from build123d import *

# Parameters (mm, degrees)
SALIENTE_EXTRUIR1_DEPTH   = 2.5
CROQUIS3_R                = 4
SALIENTE_EXTRUIR3_DEPTH   = 60
CROQUIS4_OUTSIDE_W        = 85.354
CROQUIS4_OUTSIDE_H        = 86.902
CROQUIS4_OUTSIDE_R        = 5
CORTAR_EXTRUIR1_DEPTH     = 30
CORTAR_EXTRUIR1_DRAFT     = -45
SIMETR_A1_COPY_1_SKETCH_W = 85.354
SIMETR_A1_COPY_1_SKETCH_H = 86.902
SIMETR_A1_COPY_1_SKETCH_R = 5
SIMETR_A1_COPY_1_DEPTH    = 30
SIMETR_A1_COPY_1_DRAFT    = -45


with BuildPart() as part:
    # Croquis1 → Saliente-Extruir1 (new, symmetric)
    with BuildSketch(Plane(origin=(0, 0, 0), x_dir=(1, 0, 0), z_dir=(0, 1, 0))):
        Polygon((0, -5.773502692), (5, -2.886751346), (5, 2.886751346), (0, 5.773502692), (-5, 2.886751346), (-5, -2.886751346), align=None)
    extrude(amount=SALIENTE_EXTRUIR1_DEPTH, both=True)

    # Croquis3 → Saliente-Extruir3 (add)
    with BuildSketch(Plane.XZ.offset(2.5)):
        with Locations(Location((0, 0, 0), (0, 0, 270))):
            Circle(CROQUIS3_R)
    extrude(amount=SALIENTE_EXTRUIR3_DEPTH)


with BuildPart() as cortar_extruir1_tool:
    # Croquis4 outside → Cortar-Extruir1 (with draft: the straight prism first)
    with BuildSketch(Plane.XZ.offset(2.5)):
        Rectangle(CROQUIS4_OUTSIDE_W, CROQUIS4_OUTSIDE_H)
        Circle(CROQUIS4_OUTSIDE_R, mode=Mode.SUBTRACT)
    extrude(amount=-CORTAR_EXTRUIR1_DEPTH)
    # Cortar-Extruir1: the draft: its side faces are tilted about the plane it starts from
    cortar_extruir1_sides = [cortar_extruir1_tool.faces().sort_by_distance(p)[0] for p in [
        (0, 12.5, -43.451),
        (42.677, 12.5, 0),
        (0, 12.5, 43.451),
        (-42.677, 12.5, 0),
        (-5, 12.5, 0),
    ]]
    draft(cortar_extruir1_sides, Plane.XZ.offset(2.5), CORTAR_EXTRUIR1_DRAFT)


with BuildPart() as part_1:
    add(part.part)

    # Cortar-Extruir1: cut by cortar_extruir1_tool
    add(cortar_extruir1_tool.part, mode=Mode.SUBTRACT)


with BuildPart() as simetr_a1_copy_1_tool:
    # Simetría1 copy 1 sketch → Simetría1 copy 1 (with draft: the straight prism first)
    with BuildSketch(Plane(origin=(0, 2.5, 0), x_dir=(1, 0, 0), z_dir=(0, 1, 0))):
        Rectangle(SIMETR_A1_COPY_1_SKETCH_W, SIMETR_A1_COPY_1_SKETCH_H)
        Circle(SIMETR_A1_COPY_1_SKETCH_R, mode=Mode.SUBTRACT)
    extrude(amount=-SIMETR_A1_COPY_1_DEPTH)
    # Simetría1 copy 1: the draft: its side faces are tilted about the plane it starts from
    simetr_a1_copy_1_sides = [simetr_a1_copy_1_tool.faces().sort_by_distance(p)[0] for p in [
        (0, -12.5, -43.451),
        (42.677, -12.5, 0),
        (0, -12.5, 43.451),
        (-42.677, -12.5, 0),
        (-5, -12.5, 0),
    ]]
    draft(simetr_a1_copy_1_sides, Plane(origin=(0, 2.5, 0), x_dir=(1, 0, 0), z_dir=(0, 1, 0)), SIMETR_A1_COPY_1_DRAFT)


with BuildPart() as part_2:
    add(part_1.part)

    # Simetría1 copy 1: cut by simetr_a1_copy_1_tool
    add(simetr_a1_copy_1_tool.part, mode=Mode.SUBTRACT)


solid = part_2.part
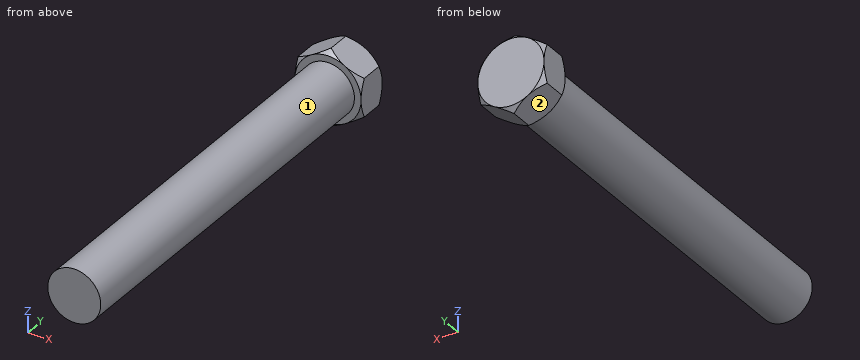
Read the model definition and answer for the solid it produces. Units are mm, in the model's axes. Face numbers are marked on the shaded views. A direction names the side the tool comes from. Round coordinates to 2 decimals unless told otherwise and drop trailing zeros. Order: outer loops, then holes, each group sorted by start corner. A loop starts at its lowest first (then second) coordinate and runs counter-clockwise, first axis right, second up.
1) Flat-ended cylindrical pins translate along their axes: pin 1 (5 mm diameter, centred on y = -26.5, z = -4, fed in from -X); pin 2 (3 mm diameter, centred on y = -43, z = 4, fed in from -X); pin 3 (1.5 mm diameter, centred on y = -9.5, z = 0, fed in from +X). Find the tip coordinate at first contact, or state that the pin passes through.
2) The part is cut by section A-A on y = -16.5. Write down the section's boundary in (x, z).
3) For the marked faces 1 and 2, determine the directions among +Z, -Z, +X, -X, +Y, -Y from which every point of the face is accessible in a straight line to the end or side of a thin tool.
4) Straight lines are drawn through the part: L1, parallel to Y at x = 1, z = 4.5; L2, parallel to Z at x = -3.5, y = -23; L3, parallel to Z at x = 0.25, y = -14. For each, find the intervals that lie inside material, in ascending order.
Resolved:
1. pin 1: stops at x = -3.71
1. pin 2: stops at x = -3.12
1. pin 3: stops at x = 4
2. outline: circle Ø8 at (0, 0)
3. face 1: -Y
3. face 2: -Z, -X, +Y, -Y
4. L1: y = -2.5 to 2.5
4. L2: z = -1.94 to 1.94
4. L3: z = -3.99 to 3.99
